Verification items for the finished model (mm, model axes). A direction names the side the tool comes from. Coordinates: 2 decimals unless noted, no trailing zeros. Loops run counter-clockwise (first coordinate to the right, second up) from the corner with the lowest first, then second, coordinate; pieces in that order, holes last.
Q1. Mould release check, pull along Y, two halves, no side actions. Record for faces 4 (the face through (-3.14, -6.03, 23.85)), 5 (the face through (-7.493, 0.33, 11.888)): +Y half, -Y half, draft (parallel to the pull), parting line (faces both ways), or undercut.
Q2. Access from +Z, -Z, +X, -X, +Y, -Y to the whole of each face (thin tool, end or side, straight path). Record for faces 1 (the face through (-0.534, 4.065, 11.832)), 2 (the face through (3.65, -2.8, 0.15)), 3 (the face through (5, 0, 23.7)).
Q3. Material ranges on probe 1 along Y at (x, z) = (0, 23.8); probe 2 along Z at (x, y) = (6.75, -3); probe 3 along X at (y, z) = (2.75, 4.25), recorded low to high.
Q4. Go/stop test with flat-tipped pins: P1, Ø7.5, axis at x = -1.5, y = 1, coming from the +Z side; P2, Ø6, axis at x = -5, z = 18, coming from the -Y side; P3, Ø5, axis at y = -5, z = 6.5, coming from the +X side; P4, Ø4, axis at y = 5.5, z = 10.5, coming from the -X side. Record where each tip stops, or that it passes through.
Q5. Sectioned sample at A-A (z = 15.75). Enter the section's corners in (x, y).
```python
from build123d import *

# Parameters (mm, degrees)
CROQUIS1_R              = 7.5
CROQUIS1_R_2            = 4.1
SALIENTE_EXTRUIR1_DEPTH = 24
CROQUIS2_W              = 0.4
CROQUIS2_H              = 1


with BuildPart() as part:
    # Croquis1 → Saliente-Extruir1 (new body)
    with BuildSketch(Plane.XY):
        Circle(CROQUIS1_R)
        Circle(CROQUIS1_R_2, mode=Mode.SUBTRACT)
    extrude(amount=SALIENTE_EXTRUIR1_DEPTH)

    # Croquis2 → Cortar-Revolución1 (revolve, cut)
    with BuildSketch(Plane(origin=(0, 0, 0), x_dir=(1, 0, 0), z_dir=(0, 1, 0))):
        Polygon((-7.5, -0.02), (-7.4, 0), (-6.8, 0), (-6.8, -0.3), (-4.6, -0.3), (-4.6, 0), (-4.1, 0), (-4.1, 0.7), (-7.5, 0.7), align=None)
        Polygon((-7.5, -24.7), (-7.5, -23.98), (-7.4, -24), (-6.8, -24), (-6.8, -23.7), (-4.6, -23.7), (-4.6, -24), (-4.1, -24), (-4.1, -24.7), align=None)
        with Locations((-7.5, -3.5)):
            Rectangle(CROQUIS2_W, CROQUIS2_H)
        with Locations((-7.5, -20.5)):
            Rectangle(CROQUIS2_W, CROQUIS2_H)
    revolve(axis=Axis((0, 0, 24), (0, 0, -1)), mode=Mode.SUBTRACT)


solid = part.part
```
Geometry check:
1. face 4: undercut
1. face 5: parting line
2. face 1: +Z, -Z
2. face 2: -Z
2. face 3: +Z
3. probe 1: y = -7.5 to -6.8, -4.6 to -4.1, 4.1 to 4.6, 6.8 to 7.5
3. probe 2: z = 0 to 3, 4 to 20, 21 to 24
3. probe 3: x = -6.98 to -3.04, 3.04 to 6.98
4. P1: stops at z = 24
4. P2: stops at y = -7.23
4. P3: stops at x = 7.07
4. P4: stops at x = -6.63
5. outline: circle Ø15 at (0, 0); hole circle Ø8.2 at (0, 0)
